```python
from build123d import *

# Parameters (mm, degrees)
SKETCH1_R               = 11
BOSS_EXTRUDE1_DEPTH     = 6.5
SKETCH2_R               = 1
CUT_EXTRUDE1_DEPTH      = 17.8597153
CIRPATTERN1_COUNT       = 4
SKETCH3_R               = 6.2
BOSS_EXTRUDE2_DEPTH     = 15
CUT_EXTRUDE2_DEPTH      = 27.537709019
CUT_EXTRUDE2_DEPTH_BACK = 27.537709019
SKETCH4_R               = 0.9


with BuildPart() as part:
    # Sketch1 → Boss-Extrude1 (new body)
    with BuildSketch(Plane(origin=(0, 0, 0), x_dir=(1, 0, 0), z_dir=(0, 1, 0))):
        with Locations(Location((0, 0, 0), (0, 0, 90))):
            Circle(SKETCH1_R)
    extrude(amount=BOSS_EXTRUDE1_DEPTH)

    # Sketch2 → Cut-Extrude1 (cut, through all)
    with BuildSketch(Plane(origin=(0, 6.5, 0), x_dir=(1, 0, 0), z_dir=(0, 1, 0))):
        with Locations(Location((0, 7.9, 0), (0, 0, 270))):
            Circle(SKETCH2_R)
    cut_extrude1 = extrude(amount=-CUT_EXTRUDE1_DEPTH, mode=Mode.SUBTRACT)

    # CirPattern1: Cut-Extrude1 ×4 about axis
    cirpattern1_axis = Axis((0, 0, 0), (0, 1, 0))
    for i in range(1, CIRPATTERN1_COUNT):
        add(cut_extrude1.rotate(cirpattern1_axis, i * 360 / CIRPATTERN1_COUNT), mode=Mode.SUBTRACT)

    # Sketch3 → Boss-Extrude2 (add)
    with BuildSketch(Plane(origin=(0, 6.5, 0), x_dir=(1, 0, 0), z_dir=(0, 1, 0))):
        with Locations(Location((0, 0, 0), (0, 0, 270))):
            Circle(SKETCH3_R)
    extrude(amount=BOSS_EXTRUDE2_DEPTH)

    # Sketch4 → Cut-Extrude2 (cut, two sides: drawn at the far end of the back side and taken through both)
    with BuildSketch(Plane(origin=(0, 0, 0), x_dir=(0, 0, -1), z_dir=(1, 0, 0)).offset(-CUT_EXTRUDE2_DEPTH_BACK)):
        with Locations((0, 14.5)):
            Circle(SKETCH4_R)
    extrude(amount=CUT_EXTRUDE2_DEPTH + CUT_EXTRUDE2_DEPTH_BACK, mode=Mode.SUBTRACT)


solid = part.part
```
The model under review builds one solid part; all positions refer to its coordinate system, in mm. A direction names the side the tool comes from. Give positions to 0.01 mm unless a question says otherwise; leave off trailing zeros. Write each loop counter-clockwise with the first axis right and the second up, starting at its lowest first coordinate (ties: lowest second). Pieces come first, ordered by that corner, then holes. Notation, with made-up numbers: (-36, 16.25) -> (11, 16.25) arc R18 cw to (11, 40.25) -> close; hole circle Ø8 at (-36.5, 5). An arc over 180 degrees is marked (long way). Answer in a Markdown table with one row per item.
1) For L1, parallel to Y at x = -1, z = 0; L2, parallel to Y at x = 4, z = -5.25; L3, parallel to Y at x = -6, z = -0.5, list the stretches that pass through material, from the lowest coordinate up. Write a range as [from, to].
Worked answers:
| item | result |
|---|---|
| L1 | [0, 13.6], [15.4, 21.5] |
| L2 | [0, 6.5] |
| L3 | [0, 13.75], [15.25, 21.5] |
2) Add section D-D on z = -7.9. State the section outline as (x, y) points, plus the area to 3 significant figures.
Worked answers:
| item | result |
|---|---|
| outline | (-7.65, 0) -> (-1, 0) -> (-1, 6.5) -> (-7.65, 6.5) -> close; (1, 0) -> (7.65, 0) -> (7.65, 6.5) -> (1, 6.5) -> close |
| area | 86.5 mm² |
3) Mouldability with a two-part tool opening along X and no side actions: class faces 1 (the cylindrical face through (-0.09, 15.39, 0.12)), 2 (the cylindrical face through (0.6, 3.3, 8.7)), 3 (the cylindrical face through (10.74, 3.2, 2.38)) as +X half, -X half, draft (parallel to the pull), parting line (faces both ways), or undercut.
Worked answers:
| item | result |
|---|---|
| face 1 | draft |
| face 2 | undercut |
| face 3 | parting line |
4) Add section A-A on x = 0. State the section outline as (y, z) points, plus the area to 3 significant figures.
Worked answers:
| item | result |
|---|---|
| outline | (0, -11) -> (6.5, -11) -> (6.5, -8.9) -> (0, -8.9) -> close; (0, -6.9) -> (6.5, -6.9) -> (6.5, -6.2) -> (21.5, -6.2) -> (21.5, 6.2) -> (6.5, 6.2) -> (6.5, 6.9) -> (0, 6.9) -> close; (0, 8.9) -> (6.5, 8.9) -> (6.5, 11) -> (0, 11) -> close; hole circle Ø1.8 at (14.5, 0) |
| area | 300 mm² |
5) Tool access review of faces 4 (the cylindrical face through (-0.6, 3.3, -8.7)), 5 (the flat face through (5, 6.5, -5)): name each direction out of +Z, -Z, +X, -X, +Y, -Y from which nothing blocks a thin tool from reaching the whole face with its end or side.
Worked answers:
| item | result |
|---|---|
| face 4 | +Y, -Y |
| face 5 | +Y |
6) Add section B-B on z = 0. State the section outline as (x, y) points.
Worked answers:
| item | result |
|---|---|
| outline | (-11, 0) -> (-8.9, 0) -> (-8.9, 6.5) -> (-11, 6.5) -> close; (-6.9, 0) -> (6.9, 0) -> (6.9, 6.5) -> (6.2, 6.5) -> (6.2, 13.6) -> (-6.2, 13.6) -> (-6.2, 6.5) -> (-6.9, 6.5) -> close; (-6.2, 15.4) -> (6.2, 15.4) -> (6.2, 21.5) -> (-6.2, 21.5) -> close; (8.9, 0) -> (11, 0) -> (11, 6.5) -> (8.9, 6.5) -> close |
7) Add section C-C on y = 3.75. State the section outline as (x, z) points, plus the area to 3 significant figures.
Worked answers:
| item | result |
|---|---|
| outline | circle Ø22 at (0, 0); hole circle Ø2 at (-7.9, 0); hole circle Ø2 at (0, -7.9); hole circle Ø2 at (0, 7.9); hole circle Ø2 at (7.9, 0) |
| area | 368 mm² |
8) Clearance check with flat-ended pins moving along their axes: P1, Ø3, axis at y = 14.5, z = 0, coming from the -X side; P2, Ø2, axis at y = 4.5, z = -7, coming from the +X side; P3, Ø2.5, axis at x = -7.9, z = 0, coming from the -Y side; P4, Ø4, axis at y = 14, z = 4.5, coming from the -X side. State where each tip first meets the part, or that it passes through.
Worked answers:
| item | result |
|---|---|
| P1 | x = -6.2 |
| P2 | x = 9.22 |
| P3 | y = 0 |
| P4 | x = -5.67 |
